Read the model definition and answer for the solid it produces. Units are mm, in the model's axes. A direction names the side the tool comes from. Coordinates: 2 decimals unless noted, no trailing zeros. Write each loop counter-clockwise with the first axis right and the second up, starting at its lowest first coordinate (ties: lowest second). Pieces come first, ordered by that corner, then holes. Notation, with made-up numbers: (-28.75, 84.5) -> (10.25, 84.5) arc R31 cw to (10.25, 118.5) -> close; hole circle Ø2 at (77, 1). An arc over 180 degrees is marked (long way). One line per item, written item: value. Start each with the question number.
1. Consider line 1 along Y through (x, z) = (33, 0.45); line 2 along Z through (x, y) = (0.5, 14.5); line 3 along X through (y, z) = (-23.5, 0.2). Determine where each line is inside the solid, lowest interval first.
2. Find section C-C, the plane x = 11.5. Write down the section's boundary in (y, z) (3 decimals), and give its area (3 significant figures).
3. For faces 4 (the flat face through (0, -16.75, 3)), 5 (the flat face through (0, 15.75, 3)), 6 (the flat face through (-24, -15.75, 3)), determine the directions among +Z, -Z, +X, -X, +Y, -Y from which every point of the face is accessible in a straight line to the end or side of a thin tool.
4. Find section B-B, the plane x = 33. Write down the section's boundary in (y, z).
5. For a pull along X with two mould halves and no side action, classify faces 1 (the flat face through (29.75, 0, 3)), 2 (the flat face through (24, -15.75, 3)), 3 (the cylindrical face through (34.19, -24.38, 0.49)) as pulls with the +X half, pulls with the -X half, needs draft (parallel to the pull), parting line crosses it, or undercut.
6. Find section D-D, the plane y = 6.5. Write down the section's boundary in (x, z) (3 decimals).
7. Find section A-A, the plane y = -24. Write down the section's boundary in (x, z), and give its area (3 significant figures).
8. Given P1, Ø1.6, axis at y = 3, z = 3, coming from the -X side; P2, Ø1.5, axis at x = -23, z = 2.5, coming from the +Y side; P3, Ø2, axis at y = 4.5, z = 2.5, coming from the +X side; P4, Ø2, axis at x = -33, y = -24, coming from the +Z side, each flat-ended and moving along its own axis, determine where each tip first touches the part or whether it passes through.
Autodesk Inventor part; units mm, degrees
ref_plane "YZ Plane" through (0, 0, 0) normal (1, 0, 0) x (0, 1, 0)
ref_plane "XZ Plane" through (0, 0, 0) normal (0, 1, 0) x (-1, 0, 0)
ref_plane "XY Plane" through (0, 0, 0) normal (0, 0, 1) x (1, 0, 0)
sketch "Sketch1" plane through (0, 0, 0) normal (0, 0, 1) x (1, 0, 0)
  line L0 (-27.505, 13.7) -> (27.505, 13.7)
  line L1 (27.505, 13.7) -> (27.505, -13.7)
  line L2 (27.505, -13.7) -> (-27.505, -13.7)
  line L3 (-27.505, -13.7) -> (-27.505, 13.7)
  line L4 (-49, 0) -> (49, 0) construction
  line L5 (0, -36) -> (0, 34) construction
  line L6 (-28.505, 14.745) -> (28.505, 14.745)
  line L7 (28.505, 14.745) -> (28.505, -14.745)
  line L8 (28.505, -14.745) -> (-28.505, -14.745)
  line L9 (-28.505, -14.745) -> (-28.505, 14.745)
  line L10 (-29.75, 15.75) -> (29.75, 15.75)
  line L11 (29.75, 15.75) -> (29.75, -15.75)
  line L12 (-29.75, -15.75) -> (-29.75, 15.75)
  line L13 (-31, 17) -> (31, 17)
  line L14 (31, 17) -> (31, -22)
  line L15 (31, -22) -> (-31, -22)
  line L16 (-31, -22) -> (-31, 17)
  line L17 (-31, 17) -> (-29.75, 15.75) construction
  line L18 (-18, -15.75) -> (-17, -16.75)
  line L19 (-17, -16.75) -> (17, -16.75)
  line L20 (17, -16.75) -> (18, -15.75)
  line L21 (29.75, -15.75) -> (18, -15.75)
  line L22 (-18, -15.75) -> (-29.75, -15.75)
  line L23 (-35, 24) -> (35, 24)
  line L24 (35, 24) -> (35, -26)
  line L25 (35, -26) -> (-35, -26)
  line L26 (-35, -26) -> (-35, 24)
  line L27 (-35, -26) -> (-31, -22) construction
  circle A0 centre (-33, -24) radius 1.25
  circle A1 centre (-33, 22) radius 1.25
  circle A2 centre (33, -24) radius 1.25
  circle A3 centre (33, 22) radius 1.25
  point P0 (0, 0)
  dimension "d0" = 55.01
  dimension "d1" = 27.4
  dimension "d2" = 57.01
  dimension "d3" = 29.49
  dimension "d4" = 59.5
  dimension "d5" = 31.5
  dimension "d6" = 62
  dimension "d7" = 39
  dimension "d8" = 34
  dimension "d10" = 1
  dimension "d11" = 70
  dimension "d12" = 50
  dimension "d21" = 2
  dimension "d22" = 2.5
  dimension "d33" = 46
  dimension "d36" = 66
extrude "Extrusion1" add sketch "Sketch1" along normal blind 1 contours L0 L1 L2 L3 | L6 L7 L8 L9 | L10 L11 L21 L20 L19 L18 L22 L12 | L13 L14 L15 L16 | L23 L24 L25 L26
extrude "Extrusion2" add sketch "Sketch1" along normal blind 2 contours L0 L1 L2 L3
extrude "Extrusion3" add sketch "Sketch1" along normal blind 2 from surface at 2 contours L0 L1 L2 L3 | L6 L7 L8 L9 | L10 L11 L21 L20 L19 L18 L22 L12
extrude "Extrusion4" add sketch "Sketch1" along normal blind 0.2 from surface at 4 contours L0 L1 L2 L3 | L6 L7 L8 L9
equation "\"d33\" = d12 - 2 * d21"
equation "\"d36\" = d11 - 2 * d21"
properties part number "Adafruit 2.4 OLED display"
Answer block:
1. line 1: y = -26 to -25.25, -22.75 to 20.75, 23.25 to 24
1. line 2: z = 0 to 1, 2 to 4.2
1. line 3: x = -35 to -34.15, -31.85 to 31.85, 34.15 to 35
2. outline: (-26, 0) -> (24, 0) -> (24, 1) -> (13.7, 1) -> (13.7, 2) -> (15.75, 2) -> (15.75, 4) -> (14.745, 4) -> (14.745, 4.2) -> (-14.745, 4.2) -> (-14.745, 4) -> (-16.75, 4) -> (-16.75, 2) -> (-13.7, 2) -> (-13.7, 1) -> (-26, 1) -> close
2. area: 148 mm2
3. face 4: +Z, +X, -X, -Y
3. face 5: +Z, +X, -X, +Y
3. face 6: +Z, -X, -Y
4. outline: (-26, 0) -> (-25.25, 0) -> (-25.25, 1) -> (-26, 1) -> close; (-22.75, 0) -> (20.75, 0) -> (20.75, 1) -> (-22.75, 1) -> close; (23.25, 0) -> (24, 0) -> (24, 1) -> (23.25, 1) -> close
5. face 1: pulls with the +X half
5. face 2: needs draft
5. face 3: undercut
6. outline: (-35, 0) -> (35, 0) -> (35, 1) -> (27.505, 1) -> (27.505, 2) -> (29.75, 2) -> (29.75, 4) -> (28.505, 4) -> (28.505, 4.2) -> (-28.505, 4.2) -> (-28.505, 4) -> (-29.75, 4) -> (-29.75, 2) -> (-27.505, 2) -> (-27.505, 1) -> (-35, 1) -> close
7. outline: (-35, 0) -> (-34.25, 0) -> (-34.25, 1) -> (-35, 1) -> close; (-31.75, 0) -> (31.75, 0) -> (31.75, 1) -> (-31.75, 1) -> close; (34.25, 0) -> (35, 0) -> (35, 1) -> (34.25, 1) -> close
7. area: 65.0 mm2
8. P1: stops at x = -29.75
8. P2: stops at y = 15.75
8. P3: stops at x = 29.75
8. P4: passes through
